from build123d import *

# Parameters (mm, degrees)
SKETCH1_W               = 330
SKETCH1_H               = 275
SKETCH1_W_2             = 305
SKETCH1_H_2             = 250
BOSS_EXTRUDE4_DEPTH     = 12
BOSS_EXTRUDE6_DEPTH     = 12.5
BOSS_EXTRUDE7_DEPTH     = 12.5
SKETCH6_R               = 15
SKETCH6_R_2             = 11
BOSS_EXTRUDE8_DEPTH     = 12.5
SKETCH7_R               = 11
CUT_EXTRUDE2_DEPTH      = 383.003996993
BOSS_EXTRUDE9_REACH     = 283.371
SKETCH8_W               = 12.5
SKETCH8_H               = 10
BOSS_EXTRUDE10_REACH    = 283.371
SKETCH9_W               = 12.5
SKETCH9_H               = 10
SKETCH10_W              = 25
SKETCH10_H              = 25
BOSS_EXTRUDE11_DEPTH    = 12.5
SKETCH12_W              = 280.956709722
SKETCH12_H              = 169.506953284
CUT_EXTRUDE3_DEPTH      = 311
CUT_EXTRUDE4_DEPTH      = 12
CUT_EXTRUDE4_DEPTH_BACK = 6.5
SKETCH13_W              = 294.886301965
SKETCH13_H              = 76.884210059


with BuildPart() as part:
    # Sketch1 → Boss-Extrude4 (new body)
    with BuildSketch(Plane(origin=(0, 0, 0), x_dir=(1, 0, 0), z_dir=(0, 1, 0))):
        Rectangle(SKETCH1_W, SKETCH1_H)
        Rectangle(SKETCH1_W_2, SKETCH1_H_2, mode=Mode.SUBTRACT)
    extrude(amount=BOSS_EXTRUDE4_DEPTH)

    # Sketch2 → Boss-Extrude6 (add)
    with BuildSketch(Plane(origin=(165, 0, 0), x_dir=(0, 0, -1), z_dir=(1, 0, 0))):
        Polygon((0, 152), (-137.5, 12), (-127.5, 12), (0, 141.818181818), (127.5, 12), (137.5, 12), align=None)
    extrude(amount=-BOSS_EXTRUDE6_DEPTH)

    # Sketch5 → Boss-Extrude7 (add)
    with BuildSketch(Plane.ZY.offset(165)):
        Polygon((0, 152), (-137.5, 12), (-127.5, 12), (0, 141.818181818), (127.5, 12), (137.5, 12), align=None)
    extrude(amount=-BOSS_EXTRUDE7_DEPTH)

    # Sketch6 → Boss-Extrude8 (add)
    with BuildSketch(Plane.ZY.offset(-152.5)):
        with Locations((0, 146.909090909)):
            Circle(SKETCH6_R)
        with Locations((0, 146.909090909)):
            Circle(SKETCH6_R_2, mode=Mode.SUBTRACT)
    extrude(amount=-BOSS_EXTRUDE8_DEPTH)

    # Sketch7 → Cut-Extrude2 (cut, through all)
    with BuildSketch(Plane.ZY.offset(-152.5)):
        with Locations((0, 146.909090909)):
            Circle(SKETCH7_R)
    extrude(amount=-CUT_EXTRUDE2_DEPTH, mode=Mode.SUBTRACT)

    # Boss-Extrude9: up to this plane
    boss_extrude9_end = Plane(origin=(0, 12, 0), z_dir=(0, -1, 0))
    # Sketch8 → Boss-Extrude9 (add, up to the surface)
    with BuildSketch(Plane(origin=(0, 69.631553319, 70.897581561), x_dir=(-1, 0, 0), z_dir=(0, -0.7007080148842544, -0.7134481606094221)), mode=Mode.PRIVATE) as boss_extrude9_sk1:
        with Locations((-158.75, 10.200513494)):
            Rectangle(SKETCH8_W, SKETCH8_H)
    boss_extrude9_tool1 = split(extrude(boss_extrude9_sk1.sketch, amount=BOSS_EXTRUDE9_REACH, mode=Mode.PRIVATE), bisect_by=boss_extrude9_end, keep=Keep.BOTH, mode=Mode.PRIVATE)
    add(boss_extrude9_tool1.solids().sort_by_distance((158.75, 76.909091, 63.75))[0])
    # Sketch8 → Boss-Extrude9 (add, up to the surface)
    with BuildSketch(Plane(origin=(0, 69.631553319, 70.897581561), x_dir=(-1, 0, 0), z_dir=(0, -0.7007080148842544, -0.7134481606094221)), mode=Mode.PRIVATE) as boss_extrude9_sk2:
        with Locations((158.75, 10.200513494)):
            Rectangle(SKETCH8_W, SKETCH8_H)
    boss_extrude9_tool2 = split(extrude(boss_extrude9_sk2.sketch, amount=BOSS_EXTRUDE9_REACH, mode=Mode.PRIVATE), bisect_by=boss_extrude9_end, keep=Keep.BOTH, mode=Mode.PRIVATE)
    add(boss_extrude9_tool2.solids().sort_by_distance((-158.75, 76.909091, 63.75))[0])

    # Boss-Extrude10: up to this plane
    boss_extrude10_end = Plane(origin=(0, 12, 0), z_dir=(0, -1, 0))
    # Sketch9 → Boss-Extrude10 (add, up to the surface)
    with BuildSketch(Plane(origin=(0, 69.631553319, -70.897581561), x_dir=(1, 0, 0), z_dir=(0, -0.7007080148842544, 0.7134481606094221)), mode=Mode.PRIVATE) as boss_extrude10_sk1:
        with Locations((-158.75, 10.200513494)):
            Rectangle(SKETCH9_W, SKETCH9_H)
    boss_extrude10_tool1 = split(extrude(boss_extrude10_sk1.sketch, amount=BOSS_EXTRUDE10_REACH, mode=Mode.PRIVATE), bisect_by=boss_extrude10_end, keep=Keep.BOTH, mode=Mode.PRIVATE)
    add(boss_extrude10_tool1.solids().sort_by_distance((-158.75, 76.909091, -63.75))[0])
    # Sketch9 → Boss-Extrude10 (add, up to the surface)
    with BuildSketch(Plane(origin=(0, 69.631553319, -70.897581561), x_dir=(1, 0, 0), z_dir=(0, -0.7007080148842544, 0.7134481606094221)), mode=Mode.PRIVATE) as boss_extrude10_sk2:
        with Locations((158.75, 10.200513494)):
            Rectangle(SKETCH9_W, SKETCH9_H)
    boss_extrude10_tool2 = split(extrude(boss_extrude10_sk2.sketch, amount=BOSS_EXTRUDE10_REACH, mode=Mode.PRIVATE), bisect_by=boss_extrude10_end, keep=Keep.BOTH, mode=Mode.PRIVATE)
    add(boss_extrude10_tool2.solids().sort_by_distance((158.75, 76.909091, -63.75))[0])

    # Sketch10 → Boss-Extrude11 (add)
    with BuildSketch(Plane(origin=(-152.5, 0, 0), x_dir=(0, 0, -1), z_dir=(1, 0, 0))):
        with Locations((0, 146.909090909)):
            Rectangle(SKETCH10_W, SKETCH10_H)
    extrude(amount=-BOSS_EXTRUDE11_DEPTH)

    # Sketch11 → Revolve1 (revolve)
    with BuildSketch(Plane.XY, mode=Mode.PRIVATE) as revolve1_sk:
        with BuildLine():
            Line((152.5, 157.909090909), (152.5, 161.909090909))
            ThreePointArc((152.5, 161.909090909), (149.508436085, 160.260408588), (146.516872171, 161.909090909))
            Line((146.516872171, 161.909090909), (146.516872171, 157.909090909))
            Line((146.516872171, 157.909090909), (152.5, 157.909090909))
        make_face()
    revolve(revolve1_sk.sketch.rotate(Axis((152.5, 146.909090909, 0), (-1, 0, 0)), 270), axis=Axis((152.5, 146.909090909, 0), (-1, 0, 0)))

    # Sketch12 → Cut-Extrude3 (cut)
    with BuildSketch(Plane.ZY.offset(165)):
        with Locations((2.978354861, 84.753476642)):
            Rectangle(SKETCH12_W, SKETCH12_H)
    extrude(amount=-CUT_EXTRUDE3_DEPTH, mode=Mode.SUBTRACT)

    # Sketch13 → Cut-Extrude4 (cut, two sides: drawn at the far end of the back side and taken through both)
    with BuildSketch(Plane.ZY.offset(-146).offset(-CUT_EXTRUDE4_DEPTH_BACK)):
        with Locations((9.943150983, 38.44210503)):
            Rectangle(SKETCH13_W, SKETCH13_H)
    extrude(amount=CUT_EXTRUDE4_DEPTH + CUT_EXTRUDE4_DEPTH_BACK, mode=Mode.SUBTRACT)


solid = part.part
Read the model definition and answer for the solid it produces. Units are mm, in the model's axes. A direction names the side the tool comes from. Round coordinates to 2 decimals unless told otherwise and drop trailing zeros. Write each loop counter-clockwise with the first axis right and the second up, starting at its lowest first coordinate (ties: lowest second). Pieces come first, ordered by that corner, then holes.
1. Given pin 1 Ø5 at (x, z) = (149, 50.5) entering from -Y; pin 2 Ø8 at (x, y) = (150, 105.5) entering from +Z; pin 3 Ø6 at (x, z) = (157.5, 87.5) entering from +Y; pin 4 Ø4 at (x, z) = (158, 57.5) entering from +Y, each flat-ended and moving along its own axis, determine where each tip first touches the part or whether it passes through.
2. The part is cut by section C-C, the plane z = 91.5. Determine the outline of the cut face in (x, y).
3. Determine the mould class of faces 3 (the face through (146.517, 157, -5)), 4 (the face through (165, 38, -22)), 5 (the face through (159, 6, 137.5)) for opening direction X: pulls with the +X half, pulls with the -X half, needs draft (parallel to the pull), parting line crosses it, or undercut.
4. The part is cut by section A-A, the plane y = 108. Determine the outline of the cut face in (x, z).
5. Straight lines are drawn through the part: L1, parallel to Z at x = 164, y = 39.5; L2, parallel to Z at x = 163.5, y = 31; L3, parallel to Y at x = 153.25, z = 46.5. For each, find the intervals that lie inside material, in ascending order.
6. Which of the six approach directions +Z, -Z, +X, -X, +Y, -Y give full straight-line access (tool end or side, diameter ignored) to faces 1 (the face through (159, 6, -137.5)), 2 (the face through (158.838, 51.305, 30.545))?
7. The part is cut by section D-D, the plane x = 155.5. Determine the outline of the cut face in (y, z).
8. The part is cut by section B-B, the plane z = -40.5. Determine the outline of the cut face in (x, y), then the cut area to 3 significant figures.
Values:
1. pin 1: passes through
1. pin 2: stops at z = 48.74
1. pin 3: stops at y = 65.96
1. pin 4: stops at y = 95.49
2. outline: (152.5, 0) - (165, 0) - (165, 12) - (152.5, 12) - close; (152.5, 48.65) - (165, 48.65) - (165, 58.84) - (152.5, 58.84) - close
3. face 3: pulls with the -X half
3. face 4: pulls with the +X half
3. face 5: needs draft
4. outline: (152.5, -43.21) - (165, -43.21) - (165, -33.21) - (152.5, -33.21) - close; (152.5, 33.21) - (165, 33.21) - (165, 43.21) - (152.5, 43.21) - close
5. L1: z = -110.49 to -100.49, -32.8 to -18.53, 18.53 to 32.8, 100.49 to 110.49
5. L2: z = -118.84 to -108.84, -24.14 to -9.87, 9.87 to 24.14, 108.84 to 118.84
5. L3: y = 0 to 12, 52.96 to 66.98, 94.47 to 104.65
6. face 1: -Z, +X, -X, +Y, -Y
6. face 2: +X, -X
7. outline: (0, -137.5) - (12, -137.5) - (139.01, -12.75) arc R15 ccw (long way) to (139.01, 12.75) - (12, 137.5) - (0, 137.5) - close; hole (12, -127.5) - (73.34, -67.25) - (14.3, -7.14) - (12, -9.47) - close; hole (12, 9.47) - (14.3, 7.14) - (73.34, 67.25) - (12, 127.5) - close; hole (21.31, 0) - (80.48, -60.25) - (134.01, -7.66) arc R15 cw to (134.01, 7.66) - (80.48, 60.25) - close; hole circle Ø22 at (146.91, 0)
8. outline: (152.5, 0) - (165, 0) - (165, 12) - (152.5, 12) - close; (152.5, 47.07) - (165, 47.07) - (165, 61.08) - (152.5, 61.08) - close; (152.5, 100.58) - (165, 100.58) - (165, 110.76) - (152.5, 110.76) - close
8. area: 452 mm2
